Autodesk Inventor part; units mm, degrees
ref_plane "YZ Plane" through (0, 0, 0) normal (1, 0, 0) x (0, 1, 0)
ref_plane "XZ Plane" through (0, 0, 0) normal (0, 1, 0) x (-1, 0, 0)
ref_plane "XY Plane" through (0, 0, 0) normal (0, 0, 1) x (1, 0, 0)
sketch "Boceto1" plane through (0, 0, 0) normal (0, 1, 0) x (-1, 0, 0)
  line L0 (27.5, 25) -> (-27.5, 25)
  line L1 (-27.5, 25) -> (-27.5, -25)
  line L2 (-27.5, -25) -> (27.5, -25)
  line L3 (27.5, -25) -> (27.5, 25)
  line L4 (27.5, 25) -> (-27.5, -25) construction
  line L5 (-27.5, 25) -> (27.5, -25) construction
  point P0 (0, 0)
  dimension "d0" = 55
  dimension "d1" = 50
extrude "Extrusión1" add sketch "Boceto1" along normal blind 3
sketch "Boceto2" plane through (0, 3, 0) normal (0, 1, 0) x (1, 0, 0)
  line L0 (10, 22) -> (-10, 22)
  line L1 (-10, 22) -> (-10, 28)
  line L2 (-10, 28) -> (10, 28)
  line L3 (10, 28) -> (10, 22)
  line L4 (27.5, 25) -> (-27.5, 25) construction
  line L5 (10, 22) -> (-10, 28) construction
  line L6 (-10, 22) -> (10, 28) construction
  point P0 (0, 0)
  point P1 (0, 25)
  dimension "d4" = 6
  dimension "d5" = 20
extrude "Extrusión2" add sketch "Boceto2" against normal blind 3
fillet "Empalme1" radius 2 4 edges at (-27.5, 1.5, -25) (-10, 1.5, -28) (10, 1.5, -28) (27.5, 1.5, -25)
sketch "Boceto3" plane through (0, 3, 0) normal (0, 1, 0) x (1, 0, 0)
  circle A0 centre (-20, 10) radius 1.6 construction
  circle A1 centre (-10, -5) radius 1.5 construction
  circle A2 centre (-10, 10) radius 1.6 construction
  line L0 (0, 38.6) -> (0, -35.6) construction
  circle A3 centre (20, 10) radius 1.6 construction
  circle A4 centre (10, 10) radius 1.6 construction
  circle A5 centre (-22, -19.2272) radius 1.7 construction
  circle A6 centre (2, -19.2272) radius 1.7 construction
  point P0 (0, 0)
hole "Agujero1" at (-20, 3, -10) at (-10, 3, -10) at (10, 3, -10) at (20, 3, -10) at (2, 3, 19.2272) at (-22, 3, 19.2272) direction (0, -1, 0) diameter 3 end through all
sketch "Boceto4" plane through (0, 3, 0) normal (0, 1, 0) x (1, 0, 0)
  circle A0 centre (-10, -5) radius 1.5 construction
  point P0 (0, 0)
hole "Agujero2" at (-10, 3, 5) direction (0, -1, 0) diameter 5.2 end through all
fillet "Empalme2" radius 12 2 edges at (27.5, 1.5, 25) (-27.5, 1.5, 25)
properties part number "PlacaBaseGarraPotenciaSTD"
CAD build for the part. Positions are in the model's coordinates, mm. A direction names the side the tool comes from. Coordinates: 2 decimals unless noted, no trailing zeros. Loops run counter-clockwise (first coordinate to the right, second up) from the corner with the lowest first, then second, coordinate; pieces in that order, holes last. Notation, with made-up numbers: (31, 53) - (55, 53) arc R25 cw to (55, 73) - close; hole circle Ø8 at (80, 87.25). An arc over 180 degrees is marked (long way). Write item = value, one per line. Start each with the question number.
Q1. Cut at C-C, the plane x = 2. List the corners of the cut face in (y, z).
Q2. Cut at B-B, the plane y = 1.7. List the corners of the cut face in (x, z), then the cut area to 3 significant figures.
Q3. Drill centre lines: L1, parallel to X at y = 1.4, z = -10; L2, parallel to X at y = 2.35, z = 19.5; L3, parallel to X at y = 0.6, z = -11. Where is each one in solid material? Low to high.
Q4. Flat gauge pins, fed straight in: pin 1 Ø1.8 at (x, z) = (-22, 19.23) entering from -Y; pin 2 Ø0.9 at (x, y) = (15, 1.5) entering from -Z; pin 3 Ø0.5 at (y, z) = (2, -25.5) entering from -X. Where does each tip first touch, or does it go through?
Q5. Cut at A-A, the plane z = 3.5. List the corners of the cut face in (x, y).
Q6. Which spindle directions (+Z, -Z, +X, -X, +Y, -Y) get a long thin tool onto all of the face, cutting with end or side? Do faces 1 (the cylindrical face through (-9.1, 1.5, -11.2)), 2 (the flat face through (-18, 1, -25)). Say none if no direction does.
Q7. Pull direction X, two halves, no side cores. Call faces 3 (the flat face through (18, 1, -25)), 4 (the cylindrical face through (10.9, 1.5, -11.2)), 5 (the cylindrical face through (-9.43, 1.48, -27.4)): pulls with the +X half, pulls with the -X half, needs draft (parallel to the pull), parting line crosses it, or undercut.
Computed:
q1.outline = (0, -28) - (3, -28) - (3, 17.73) - (0, 17.73) - close; (0, 20.73) - (3, 20.73) - (3, 25) - (0, 25) - close
q2.outline = (-27.5, -23) arc R2 ccw to (-25.5, -25) - (-10, -25) - (-10, -26) arc R2 ccw to (-8, -28) - (8, -28) arc R2 ccw to (10, -26) - (10, -25) - (25.5, -25) arc R2 ccw to (27.5, -23) - (27.5, 13) arc R12 ccw to (15.5, 25) - (-15.5, 25) arc R12 ccw to (-27.5, 13) - close; hole circle Ø3 at (-22, 19.23); hole circle Ø3 at (-20, -10); hole circle Ø5.2 at (-10, 5); hole circle Ø3 at (-10, -10); hole circle Ø3 at (2, 19.23); hole circle Ø3 at (10, -10); hole circle Ø3 at (20, -10)
q2.area = 2,680 mm²
q3.L1 = -27.5 to -21.5, -18.5 to -11.5, -8.5 to 8.5, 11.5 to 18.5, 21.5 to 27.5
q3.L2 = -25.59 to -23.47, -20.53 to 0.53, 3.47 to 25.59
q3.L3 = -27.5 to -21.12, -18.88 to -11.12, -8.88 to 8.88, 11.12 to 18.88, 21.12 to 27.5
q4.pin_1 = through
q4.pin_2 = -25
q4.pin_3 = -10
q5.outline = (-27.5, 0) - (-12.12, 0) - (-12.12, 3) - (-27.5, 3) - close; (-7.88, 0) - (27.5, 0) - (27.5, 3) - (-7.88, 3) - close
q6.face_1 = +Y, -Y
q6.face_2 = -Z, -X, +Y, -Y
q7.face_3 = needs draft
q7.face_4 = undercut
q7.face_5 = pulls with the -X half
